from build123d import *

# Parameters (mm, degrees)
SKETCH1_R           = 3.05
BOSS_EXTRUDE1_DEPTH = 2.4
SKETCH2_OUTSIDE_W   = 9.89
SKETCH2_OUTSIDE_H   = 9.89
CUT_EXTRUDE1_DEPTH  = 2.4
M3_TAPPED_HOLE1_D   = 2.5
CHAMFER1_SIZE       = 0.25


with BuildPart() as part:
    # Sketch1 → Boss-Extrude1 (new body)
    with BuildSketch(Plane(origin=(0, 0, 0), x_dir=(1, 0, 0), z_dir=(0, 1, 0))):
        with Locations(Location((0, 0, 0), (0, 0, 270))):
            Circle(SKETCH1_R)
    extrude(amount=BOSS_EXTRUDE1_DEPTH)

    # Sketch2 outside → Cut-Extrude1 (cut)
    with BuildSketch(Plane(origin=(0, 2.4, 0), x_dir=(1, 0, 0), z_dir=(0, 1, 0))):
        Rectangle(SKETCH2_OUTSIDE_W, SKETCH2_OUTSIDE_H)
        Polygon((1.58771324, 2.75), (-1.58771324, 2.75), (-3.175426481, 0), (-1.58771324, -2.75), (1.58771324, -2.75), (3.175426481, 0), align=None, mode=Mode.SUBTRACT)
    extrude(amount=-CUT_EXTRUDE1_DEPTH, mode=Mode.SUBTRACT)

    # Sketch3 → Cut-Revolve1 (revolve, cut)
    with BuildSketch(Plane(origin=(0, 0, 0), x_dir=(0, 0, -1), z_dir=(1, 0, 0))):
        Polygon((2.75, 2.4), (4, 2.4), (4, 1.678312164), align=None)
        Polygon((4, 0), (2.75, 0), (4, 0.721687836), align=None)
    revolve(axis=Axis((0, 0, 0), (0, 1, 0)), mode=Mode.SUBTRACT)

    # M3 Tapped Hole1 (through all)
    with Locations(Plane(origin=(0, 2.4, 0), x_dir=(1, 0, 0), z_dir=(0, 1, 0))):
        with Locations((0, 0)):
            Hole(M3_TAPPED_HOLE1_D / 2)

    # Chamfer1
    chamfer1_edges = [part.edges().sort_by_distance(p)[0] for p in [
        (1.25, 2.4, 0),
        (1.25, 0, 0),
    ]]
    chamfer(chamfer1_edges, length=CHAMFER1_SIZE)


solid = part.part
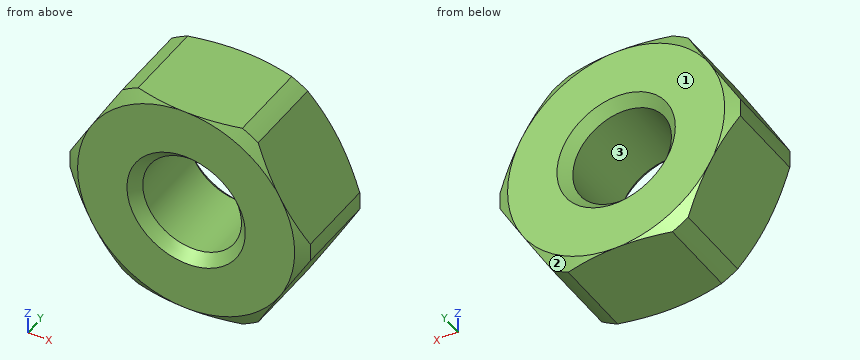
Model file for the job. Use its own axes, mm. Face numbers are marked on the shaded views. Round coordinates to 2 decimals unless told otherwise and drop trailing zeros. Order: outer loops, then holes, each group sorted by start corner. A loop starts at its lowest first (then second) coordinate and runs counter-clockwise, first axis right, second up.
(1) Band-saw the part on A-A (z = 0). List the corners of the cut face in (x, y).
(2) Drill centre lines: line 1 (X direction, y = 0.35, z = 0); line 2 (Z direction, x = 0, y = 1.8); line 3 (X direction, y = 1.7, z = -1.05). Where is each one in solid material? Low to high.
(3) Band-saw the part on B-B (y = 1.8). List the corners of the cut face in (x, z).
(4) Pull direction Z, two halves, no side cores. Call the marked faces 1, 2 and 3: released by +Z, released by -Z, zero draft, split by the parting line, or undercut.
Verdict:
1. outline: (-3.05, 0.17) - (-2.75, 0) - (-1.5, 0) - (-1.25, 0.25) - (-1.25, 2.15) - (-1.5, 2.4) - (-2.75, 2.4) - (-3.05, 2.23) - close; (1.25, 0.25) - (1.5, 0) - (2.75, 0) - (3.05, 0.17) - (3.05, 2.23) - (2.75, 2.4) - (1.5, 2.4) - (1.25, 2.15) - close
2. line 1: x = -3.05 to -1.25, 1.25 to 3.05
2. line 2: z = -2.75 to -1.25, 1.25 to 2.75
2. line 3: x = -2.57 to -0.68, 0.68 to 2.57
3. outline: (-3.04, -0.23) - (-1.72, -2.52) arc R3.05 ccw to (-1.32, -2.75) - (1.32, -2.75) arc R3.05 ccw to (1.72, -2.52) - (3.04, -0.23) arc R3.05 ccw to (3.04, 0.23) - (1.72, 2.52) arc R3.05 ccw to (1.32, 2.75) - (-1.32, 2.75) arc R3.05 ccw to (-1.72, 2.52) - (-3.04, 0.23) arc R3.05 ccw to start; hole circle Ø2.5 at (0, 0)
4. face 1: zero draft
4. face 2: released by -Z
4. face 3: undercut
